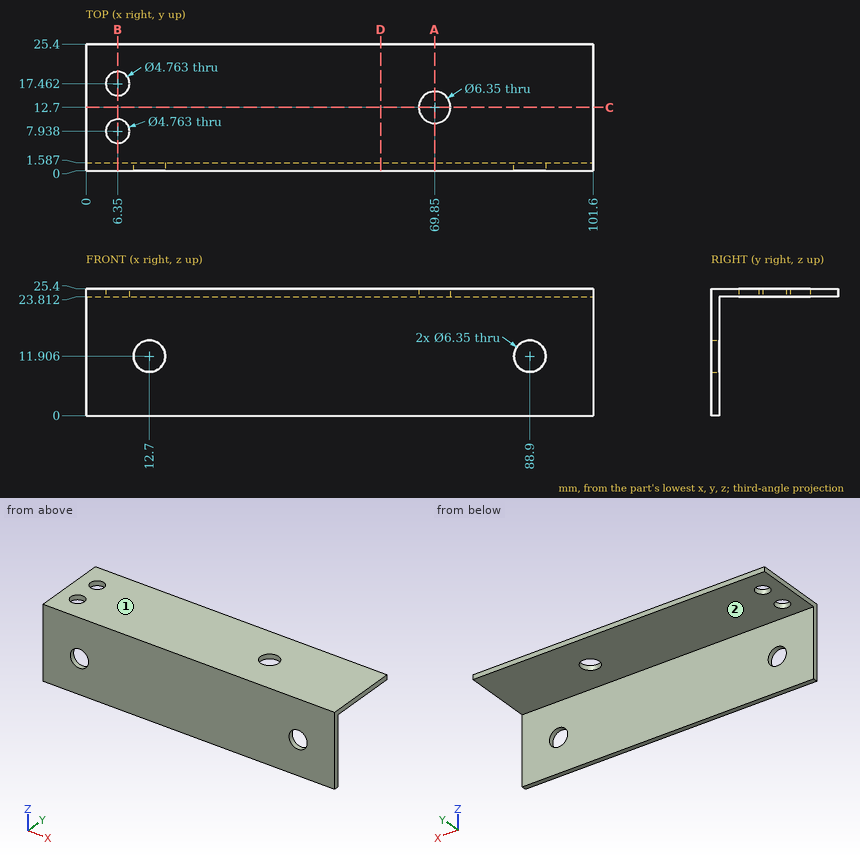
Print and shaded views of the part. All mm, measured from the part's lowest x, y and z. A direction names the side the tool comes from. Coordinates: 2 decimals unless noted, no trailing zeros. Order: outer loops, then holes, each group sorted by start corner. A loop starts at its lowest first (then second) coordinate and runs counter-clockwise, first axis right, second up. Notation, with made-up numbers: M 56,36.5 L 84,36.5 A21 ccw 84,55.5 Z; hole C -20.75,-21.5 d9. An arc over 180 degrees is marked long. One line per question, with ' | ' between items. Start each with the question number.
Q1. Saw through at D-D (x = 59). List the corners of the cut face in (y, z).
Q2. Saw through at B-B (x = 6.35). List the corners of the cut face in (y, z).
Q3. Flat gauge pins, fed straight in: pin 1 Ø12 at (x, z) = (48.5, 20) entering from +Y; pin 2 Ø10 at (x, z) = (12.7, 11.91) entering from +Y; pin 3 Ø7 at (x, y) = (64.5, 11.5) entering from -Z; pin 4 Ø4 at (x, y) = (6.35, 17.46) entering from +Z. Where does each tip first touch, or does it go through?
Q4. Saw through at A-A (x = 69.85). List the corners of the cut face in (y, z) (1 decimal).
Q5. 3-axis set-ups, long thin cutter, end or side, ignore diameter. For the marked faces 1 and 2: which of +Z, -Z, +X, -X, +Y, -Y reach the whole face in a straight line?
Q6. Saw through at C-C (y = 12.7). List the corners of the cut face in (x, z) (1 decimal).
Q7. Probe L1, parallel to Y at x = 6.35, z = 24.5; L2, parallel to Z at x = 12.7, y = 1.2; L3, parallel to Z at x = 52.5, y = 22.5. List the from-to ranges inside material, lowest first. Write a range as from..to.
Check values:
1) outline: M 0,0 L 1.59,0 L 1.59,23.81 L 25.4,23.81 L 25.4,25.4 L 0,25.4 Z
2) outline: M 0,0 L 1.59,0 L 1.59,23.81 L 5.56,23.81 L 5.56,25.4 L 0,25.4 Z; M 10.32,23.81 L 15.08,23.81 L 15.08,25.4 L 10.32,25.4 Z; M 19.84,23.81 L 25.4,23.81 L 25.4,25.4 L 19.84,25.4 Z
3) pin 1: stops at y = 25.4 | pin 2: stops at y = 1.59 | pin 3: stops at z = 23.81 | pin 4: passes through
4) outline: M 0,0 L 1.6,0 L 1.6,23.8 L 9.5,23.8 L 9.5,25.4 L 0,25.4 Z; M 15.9,23.8 L 25.4,23.8 L 25.4,25.4 L 15.9,25.4 Z
5) face 1: +Z, +X, -X, +Y, -Y | face 2: -Z, +X, -X, +Y
6) outline: M 0,23.8 L 66.7,23.8 L 66.7,25.4 L 0,25.4 Z; M 73,23.8 L 101.6,23.8 L 101.6,25.4 L 73,25.4 Z
7) L1: y = 0..5.56, 10.32..15.08, 19.84..25.4 | L2: z = 0..8.73, 15.08..25.4 | L3: z = 23.81..25.4
